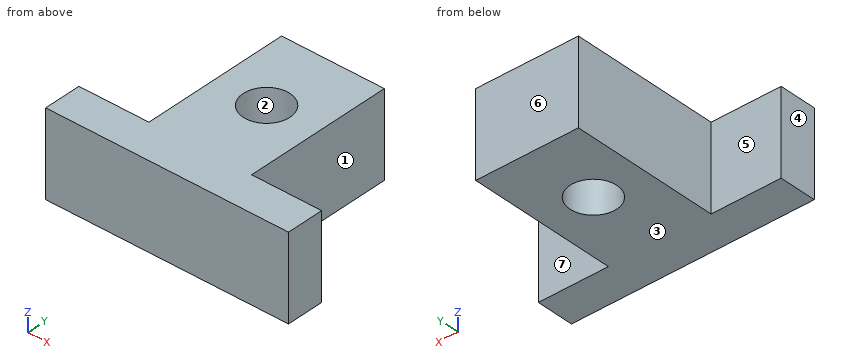
from build123d import *

# Parameters (mm, degrees)
SKETCH1_W           = 41.275
SKETCH1_H           = 6.35
SKETCH1_W_2         = 17.4625
SKETCH1_H_2         = 25.4
SKETCH1_R           = 3.96875
BOSS_EXTRUDE1_DEPTH = 14.2875


with BuildPart() as part:
    # Sketch1 → Boss-Extrude1 (new body)
    # profile 1 of 2: a face of its own
    with BuildSketch(Plane.XY):
        Rectangle(SKETCH1_W, SKETCH1_H)
    # profile 2 of 2: a face of its own
    with BuildSketch(Plane.XY):
        with Locations((0, 15.875)):
            Rectangle(SKETCH1_W_2, SKETCH1_H_2)
        with Locations((0, 15.875)):
            Circle(SKETCH1_R, mode=Mode.SUBTRACT)
    extrude(amount=BOSS_EXTRUDE1_DEPTH)


solid = part.part
For this review, take the finished solid that the model builds, in its own axes (mm). Face numbers are marked on the shaded views. A direction names the side the tool comes from. Coordinates: 2 decimals unless noted, no trailing zeros. Order: outer loops, then holes, each group sorted by start corner. A loop starts at its lowest first (then second) coordinate and runs counter-clockwise, first axis right, second up. Notation, with made-up numbers: (-6.5, 39.25) - (30.5, 39.25) arc R18 ccw to (30.5, 64.25) - close; hole circle Ø10 at (58.25, 60). An arc over 180 degrees is marked (long way). Use one line per item in the form item = value.
Q1. For probe 1 along Y at (x, z) = (0, 4.5) (3 decimals); probe 2 along Y at (x, z) = (18, 10.25) (3 decimals); probe 3 along X at (y, z) = (25, 9.5), list the stretches that pass through material, from the lowest coordinate up. Write a range as from..to.
Checked values:
probe_1 = -3.175..11.906, 19.844..28.575
probe_2 = -3.175..3.175
probe_3 = -8.73..8.73
Q2. Consider section A-A (x = 0). Give the boundary of the cut face in (y, z) (1 decimal).
Checked values:
outline = (-3.2, 0) - (11.9, 0) - (11.9, 14.3) - (-3.2, 14.3) - close; (19.8, 0) - (28.6, 0) - (28.6, 14.3) - (19.8, 14.3) - close
Q3. For the marked faces 5, 6 and 7, list the 3-axis set-ups (+Z, -Z, +X, -X, +Y, -Y) from which the entire face can be reached by the end or side of a thin tool; tool diameter is ignored.
Checked values:
face_5 = +Z, -Z, -X, +Y
face_6 = +Z, -Z, +X, -X, +Y
face_7 = +Z, -Z, +X, +Y
Q4. Consider section C-C (y = 26.5). Give the boundary of the cut face in (x, z).
Checked values:
outline = (-8.73, 0) - (8.73, 0) - (8.73, 14.29) - (-8.73, 14.29) - close
Q5. For P1, Ø2, axis at y = 17, z = 10.5, coming from the -X side; P2, Ø8, axis at x = 11.5, z = 11, coming from the +Y side (3 decimals); P3, Ø6, axis at x = -12, y = 9.5, coming from the -Z side; P4, Ø6, axis at x = -17.5, z = 4.5, coming from the +Y side (3 decimals), all flat-tipped, find the tip position at first contact; note any pin that passes through.
Checked values:
P1 = -8.73
P2 = 28.575
P3 = through
P4 = 3.175
Q6. Consider section B-B (z = 11.25). Give the boundary of the cut face in (x, y) (1 decimal).
Checked values:
outline = (-20.6, -3.2) - (20.6, -3.2) - (20.6, 3.2) - (8.7, 3.2) - (8.7, 28.6) - (-8.7, 28.6) - (-8.7, 3.2) - (-20.6, 3.2) - close; hole circle Ø7.9 at (0, 15.9)
Q7. Draft analysis for pull direction X (two halves, no side actions). For the marked faces 1, 2, 3 and 4, state which applies: +X half, -X half, draft (parallel to the pull), parting line (faces both ways), or undercut.
Checked values:
face_1 = +X half
face_2 = undercut
face_3 = draft
face_4 = -X half
